Study the drawing (mm; zero at the part's minimum x, y, z) and answer. A direction names the side the tool comes from. Coordinates: 2 decimals unless noted, no trailing zeros. Write each loop counter-clockwise with the first axis right and the second up, starting at its lowest first coordinate (ties: lowest second). Pieces come first, ordered by that corner, then holes. Notation, with made-up numbers: M -20.5,54 L 37.5,54 A8 cw 37.5,62 Z; hole C -23.75,52.25 d7. An arc over 180 degrees is marked long. Answer as CSV lines item,"result". Start each with the question number.
(1) A flat-ended cylindrical pin translates along its axis: P1, Ø1, axis at y = 14, z = 8, coming from the -X side. Find the tip coordinate at first contact, or state that the pin passes through.
(2) Find the intervals of material crossed by L1, parallel to Y at x = 2.5, z = 3; L2, parallel to Z at x = 13, y = 39; L3, parallel to X at y = 23, z = 6.75, in increasing order. Write a range as [from, to].
(3) For the marked faces 1 and 2, determine the directions among +Z, -Z, +X, -X, +Y, -Y from which every point of the face is accessible in a straight line to the end or side of a thin tool.
(4) A cutting plane is placed at D-D on y = 43. Give the vertices of the cut face in (x, z).
(5) A cutting plane is placed at B-B on y = 25. Give the vertices of the cut face in (x, z).
(6) A cutting plane is placed at C-C on x = 9. Give the vertices of the cut face in (y, z).
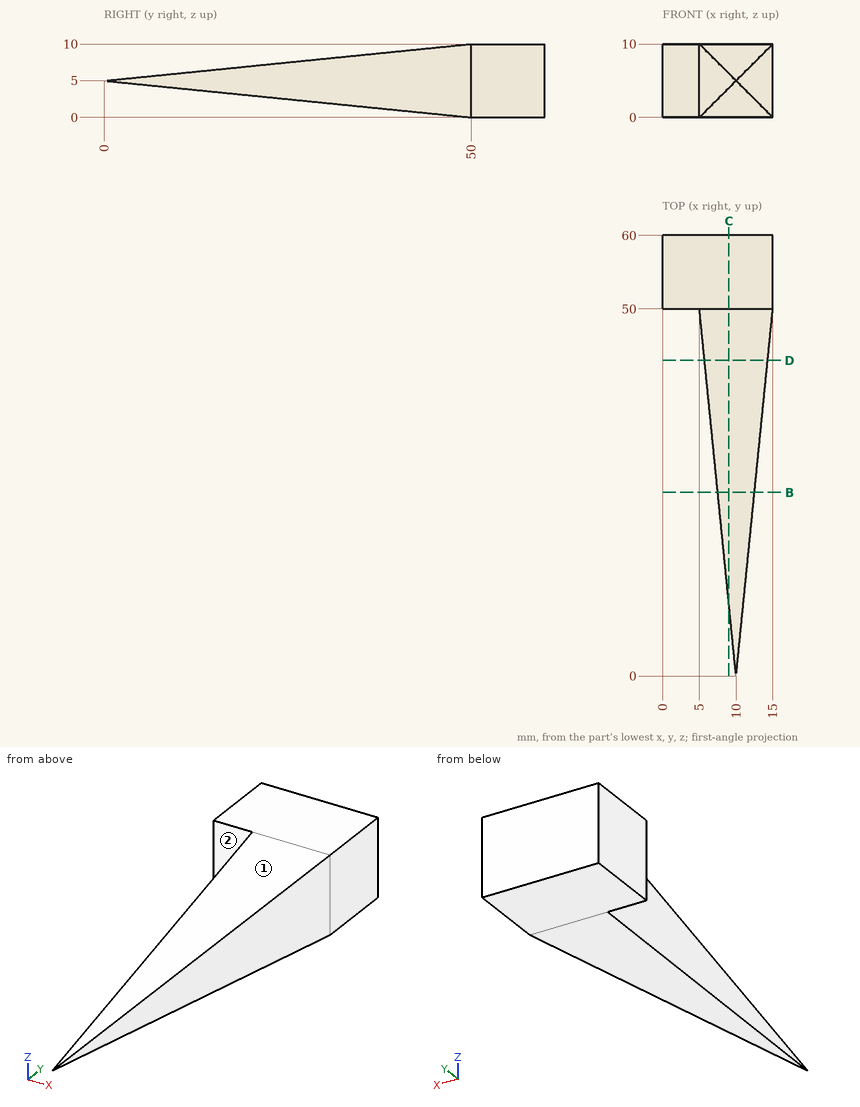
Here are the results:
1,P1,"passes through"
2,L1,"y = [50, 60]"
2,L2,"z = [1.1, 8.9]"
2,L3,"x = [7.7, 12.3]"
3,face 1,"+Z, +X, -X, -Y"
3,face 2,"+Z, -Z, -X, -Y"
4,outline,"M 5.7,0.7 L 14.3,0.7 L 14.3,9.3 L 5.7,9.3 Z"
5,outline,"M 7.5,2.5 L 12.5,2.5 L 12.5,7.5 L 7.5,7.5 Z"
6,outline,"M 10,4 L 50,0 L 60,0 L 60,10 L 50,10 L 10,6 Z"
